For this review, use the dimensioned drawing (mm, ordinates from the lowest corner) and the shaded views. A direction names the side the tool comes from. Coordinates: 2 decimals unless noted, no trailing zeros. Loops run counter-clockwise (first coordinate to the right, second up) from the corner with the lowest first, then second, coordinate; pieces in that order, holes last.
1. Take a section at C-C, the plane z = 28. State the section outline as (x, y) points.
2. Take a section at A-A, the plane y = 30. State the section outline as (x, z) points, then the cut area to 3 significant figures.
3. Clearance check with flat-ended pins moving along their axes: P1, Ø18, axis at y = 34, z = 11.5, coming from the -X side; P2, Ø4.5, axis at x = 7.5, z = 28, coming from the -Y side; P3, Ø2, axis at y = 35, z = 18.5, coming from the +X side; P4, Ø8, axis at x = 48.5, z = 5.5, coming from the -Y side. State where each tip first meets the part, or that it passes through.
4. To check wall thickness, follow probe 1 along X at (y, z) = (2, 28); probe 2 along X at (y, z) = (12, 3); probe 3 along X at (y, z) = (2, 20). State the ranges of each line that lie inside material, in increasing order.
5. Take a section at B-B, the plane x = 7.5. State the section outline as (y, z) points.
6. Take a section at D-D, the plane z = 33. State the section outline as (x, y) points.
7. Machinability: for the marked faces 1, 2 and 3, which of the approach directions +Z, -Z, +X, -X, +Y, -Y give a long, thin tool a straight path to every point of the face, cutting with its end or side? Answer none if there is none.
8. Mouldability with a two-part tool opening along X and no side actions: class the marked faces 4, 5 and 6 as pulls with the +X half, pulls with the -X half, needs draft (parallel to the pull), parting line crosses it, or undercut.
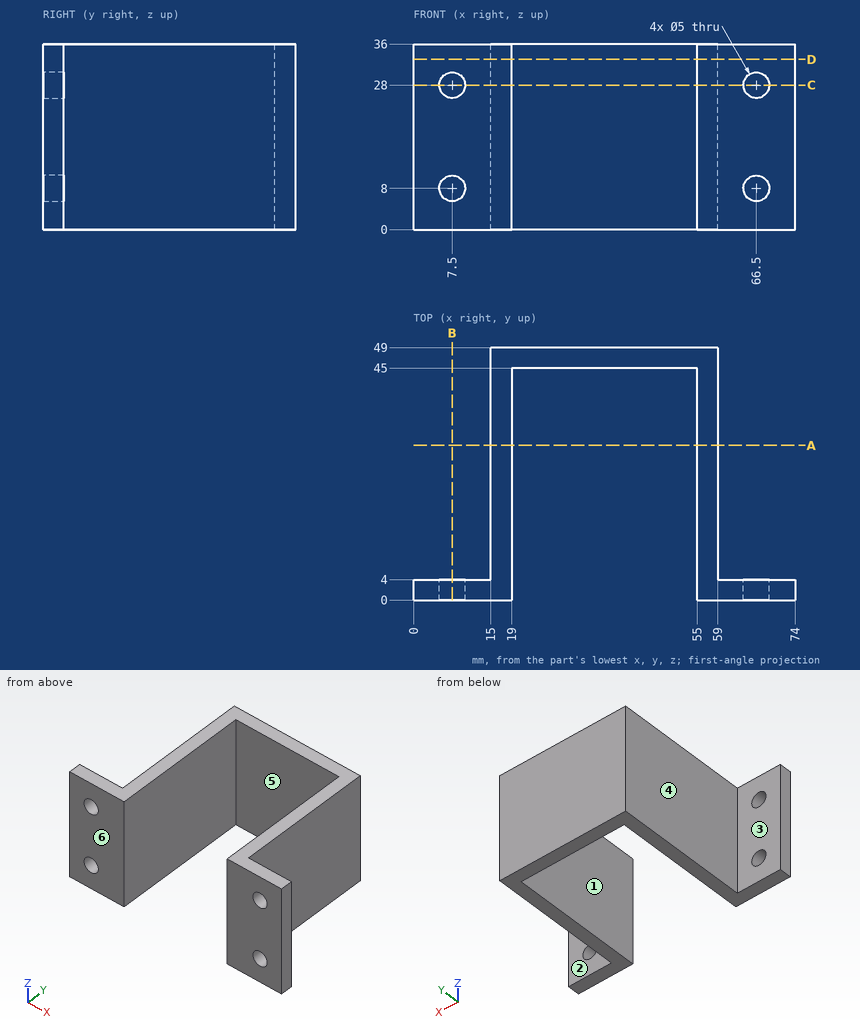
Results list:
1. outline: (0, 0) - (5, 0) - (5, 4) - (0, 4) - close; (10, 0) - (19, 0) - (19, 45) - (55, 45) - (55, 0) - (64, 0) - (64, 4) - (59, 4) - (59, 49) - (15, 49) - (15, 4) - (10, 4) - close; (69, 0) - (74, 0) - (74, 4) - (69, 4) - close
2. outline: (15, 0) - (19, 0) - (19, 36) - (15, 36) - close; (55, 0) - (59, 0) - (59, 36) - (55, 36) - close
2. area: 288 mm2
3. P1: stops at x = 15
3. P2: passes through
3. P3: stops at x = 59
3. P4: stops at y = 45
4. probe 1: x = 0 to 5, 10 to 19, 55 to 64, 69 to 74
4. probe 2: x = 15 to 19, 55 to 59
4. probe 3: x = 0 to 19, 55 to 74
5. outline: (0, 0) - (4, 0) - (4, 5.5) - (0, 5.5) - close; (0, 10.5) - (4, 10.5) - (4, 25.5) - (0, 25.5) - close; (0, 30.5) - (4, 30.5) - (4, 36) - (0, 36) - close
6. outline: (0, 0) - (19, 0) - (19, 45) - (55, 45) - (55, 0) - (74, 0) - (74, 4) - (59, 4) - (59, 49) - (15, 49) - (15, 4) - (0, 4) - close
7. face 1: +Z, -Z, -Y
7. face 2: +Z, -Z, +X, +Y
7. face 3: +Z, -Z, -X, +Y
8. face 4: pulls with the -X half
8. face 5: undercut
8. face 6: needs draft
